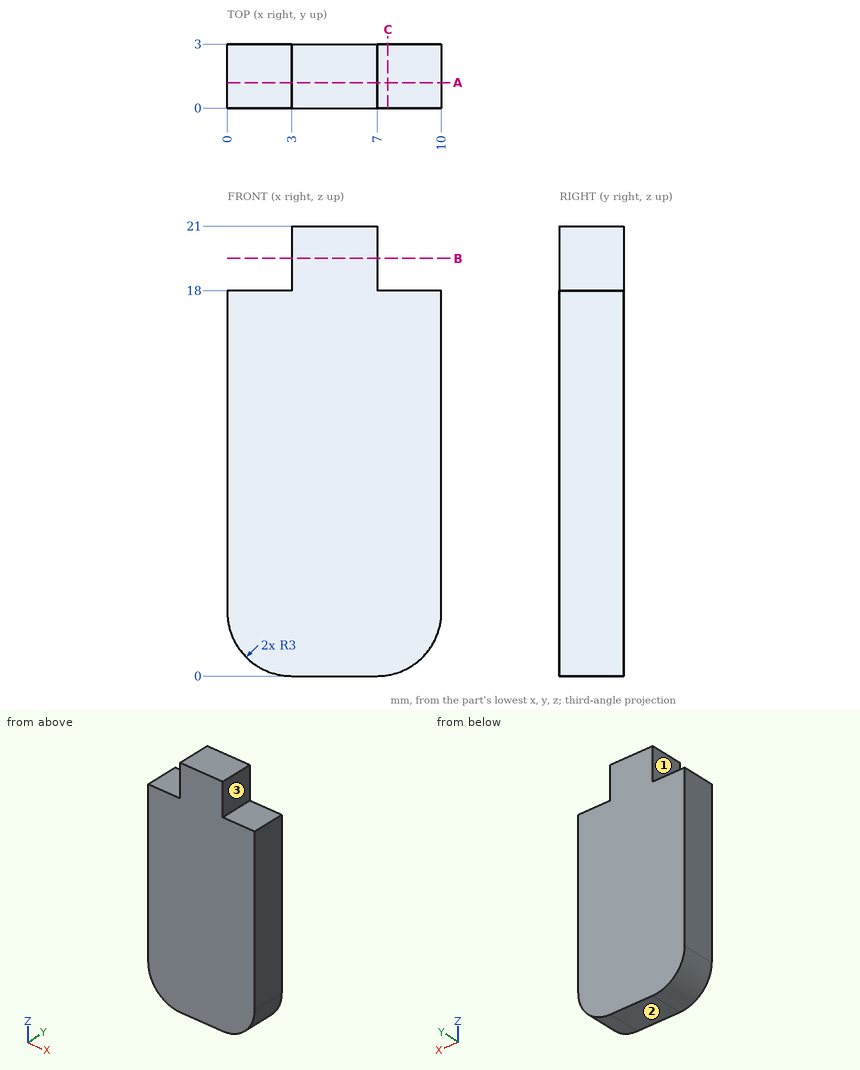
Verification items for this drawing (mm, ordinates from the low corner). A direction names the side the tool comes from. Coordinates: 2 decimals unless noted, no trailing zeros. Write each loop counter-clockwise with the first axis right and the second up, starting at its lowest first coordinate (ties: lowest second). Pieces come first, ordered by that corner, then holes. Notation, with made-up numbers: (45.5, 5.25) -> (100.5, 5.25) arc R13 cw to (100.5, 15.25) -> close; hole circle Ø3 at (24.5, 36.5). An arc over 180 degrees is marked (long way). Use CSV: the item, a comma, the result in double quotes. Start each with the question number.
Item 1: Depth check by flat-ended pin: pin 1 Ø1.5 at (x, y) = (8, 2) entering from +Z; pin 2 Ø0.9 at (y, z) = (2, 19.5) entering from -X; pin 3 Ø1.5 at (x, y) = (1.5, 2) entering from -Z; pin 4 Ø4 at (x, z) = (1, 13.5) entering from -Y. Enter the tip coordinate at first touch or a pass-through.
Item 2: Thickness scan on line 1 (X direction, y = 0.4, z = 19.25); line 2 (Z direction, x = 9.5, y = 1.4); line 3 (Z direction, x = 8.75, y = 0.85). Record the ranges inside material, lowest first.
Item 3: Cross-section at B-B, the plane z = 19.5. Record the cut outline in (x, y).
Item 4: Cross-section at A-A, the plane y = 1.2. Record the cut outline in (x, z), plus the area to 3 significant figures.
Item 5: Cross-section at C-C, the plane x = 7.5. Record the cut outline in (y, z).
Item 6: Set-up check for the marked faces 1, 2 and 3: record each of +Z, -Z, +X, -X, +Y, -Y from which the full face is reachable in a straight line by a thin tool's end or side.
Answers:
1,pin 1,"z = 18"
1,pin 2,"x = 3"
1,pin 3,"z = 0.1"
1,pin 4,"y = 0"
2,line 1,"3 to 7"
2,line 2,"1.34 to 18"
2,line 3,"0.56 to 18"
3,outline,"(3, 0) -> (7, 0) -> (7, 3) -> (3, 3) -> close"
4,outline,"(0, 3) arc R3 ccw to (3, 0) -> (7, 0) arc R3 ccw to (10, 3) -> (10, 18) -> (7, 18) -> (7, 21) -> (3, 21) -> (3, 18) -> (0, 18) -> close"
4,area,"188 mm^2"
5,outline,"(0, 0.04) -> (3, 0.04) -> (3, 18) -> (0, 18) -> close"
6,face 1,"+Z, -X, +Y, -Y"
6,face 2,"-Z, +X, -X, +Y, -Y"
6,face 3,"+Z, +X, +Y, -Y"
